```python
from build123d import *

# Parameters (mm, degrees)
SKETCH1_W           = 47
SKETCH1_H           = 78
SKETCH1_W_2         = 43
SKETCH1_H_2         = 74
EXTRUDE_THIN1_DEPTH = 15
SKETCH6_W           = 47
SKETCH6_H           = 78
BOSS_EXTRUDE1_DEPTH = 2
SKETCH8_W           = 43
SKETCH8_H           = 31
CUT_EXTRUDE1_DEPTH  = 10
CUT_EXTRUDE2_DEPTH  = 10
CUT_EXTRUDE3_DEPTH  = 10
CIRPATTERN1_COUNT   = 4
SKETCH12_R          = 1.6
CUT_EXTRUDE4_DEPTH  = 10
FILLET1_R           = 2


with BuildPart() as part:
    # Sketch1 → Extrude-Thin1 (new body)
    with BuildSketch(Plane.XY):
        with Locations((55.076537335, -3.402525622)):
            Rectangle(SKETCH1_W, SKETCH1_H)
        with Locations((55.076537335, -3.402525622)):
            Rectangle(SKETCH1_W_2, SKETCH1_H_2, mode=Mode.SUBTRACT)
    extrude(amount=EXTRUDE_THIN1_DEPTH)

    # Sketch6 → Boss-Extrude1 (add)
    with BuildSketch(Plane.XY.offset(15)):
        with Locations((55.076537335, -3.402525622)):
            Rectangle(SKETCH6_W, SKETCH6_H)
    extrude(amount=BOSS_EXTRUDE1_DEPTH)

    # Sketch8 → Cut-Extrude1 (cut)
    with BuildSketch(Plane(origin=(0, 0, 15), x_dir=(-1, 0, 0), z_dir=(0, 0, -1))):
        with Locations((-55.076537335, 18.097474378)):
            Rectangle(SKETCH8_W, SKETCH8_H)
    extrude(amount=-CUT_EXTRUDE1_DEPTH, mode=Mode.SUBTRACT)

    # Sketch9 → Cut-Extrude2 (cut)
    with BuildSketch(Plane(origin=(0, 0, 15), x_dir=(-1, 0, 0), z_dir=(0, 0, -1))):
        with BuildLine():
            ThreePointArc((-43.076537335, -18.902525622), (-43.989982945, -14.310324434), (-46.591255961, -10.417244248))
            Line((-46.591255961, -10.417244248), (-63.56181871, -27.387806996))
            ThreePointArc((-63.56181871, -27.387806996), (-50.484336147, -29.989080012), (-43.076537335, -18.902525622))
        make_face()
        with BuildLine():
            Line((-63.56181871, -27.387806996), (-46.591255961, -10.417244248))
            ThreePointArc((-46.591255961, -10.417244248), (-63.56181871, -10.417244248), (-63.56181871, -27.387806996))
        make_face()
    extrude(amount=-CUT_EXTRUDE2_DEPTH, mode=Mode.SUBTRACT)

    # Sketch11 → Cut-Extrude3 (cut)
    with BuildSketch(Plane(origin=(0, 0, 15), x_dir=(-1, 0, 0), z_dir=(0, 0, -1))):
        with BuildLine():
            ThreePointArc((-38.069685624, -3.395673911), (-38.183866325, -2.821648762), (-38.509025452, -2.335013739))
            Line((-38.509025452, -2.335013739), (-40.630345796, -4.456334083))
            ThreePointArc((-40.630345796, -4.456334083), (-38.995660475, -4.78149321), (-38.069685624, -3.395673911))
        make_face()
        with BuildLine():
            Line((-40.630345796, -4.456334083), (-38.509025452, -2.335013739))
            ThreePointArc((-38.509025452, -2.335013739), (-40.630345796, -2.335013739), (-40.630345796, -4.456334083))
        make_face()
    cut_extrude3 = extrude(amount=-CUT_EXTRUDE3_DEPTH, mode=Mode.SUBTRACT)

    # CirPattern1: Cut-Extrude3 ×4 about axis
    cirpattern1_axis = Axis((55.076537335, -18.902525622, 0), (0, 0, 1))
    for i in range(1, CIRPATTERN1_COUNT):
        add(cut_extrude3.rotate(cirpattern1_axis, i * 360 / CIRPATTERN1_COUNT), mode=Mode.SUBTRACT)

    # Sketch12 → Cut-Extrude4 (cut)
    with BuildSketch(Plane(origin=(0, 35.597474378, 0), x_dir=(1, 0, 0), z_dir=(0, 1, 0))):
        with BuildLine():
            ThreePointArc((55.076537335, -5.875), (52.451537335, -8.5), (55.076537335, -11.125))
            Line((55.076537335, -11.125), (55.076537335, -5.875))
        make_face()
        with BuildLine():
            Line((55.076537335, -5.875), (55.076537335, -11.125))
            ThreePointArc((55.076537335, -11.125), (56.932692636, -10.356155301), (57.701537335, -8.5))
            ThreePointArc((57.701537335, -8.5), (56.932692636, -6.643844699), (55.076537335, -5.875))
        make_face()
        with Locations(Location((43.446537335, -8.5, 0), (0, 0, 270))):
            Circle(SKETCH12_R)
        with Locations(Location((66.706537335, -8.5, 0), (0, 0, 270))):
            Circle(SKETCH12_R)
    extrude(amount=-CUT_EXTRUDE4_DEPTH, mode=Mode.SUBTRACT)

    # Fillet1
    fillet1_edges = [part.edges().sort_by_distance(p)[0] for p in [
        (33.576537335, 33.597474378, 8.5),
        (76.576537335, 33.597474378, 8.5),
    ]]
    fillet(fillet1_edges, radius=FILLET1_R)


solid = part.part
```
Geometry: final body of the model. Coordinates: model frame, mm. A direction names the side the tool comes from. Coordinates: 2 decimals unless noted, no trailing zeros. Loops run counter-clockwise (first coordinate to the right, second up) from the corner with the lowest first, then second, coordinate; pieces in that order, holes last. Notation, with made-up numbers: (59, 50.5) -> (115, 50.5) arc R14 cw to (115, 57.5) -> close; hole circle Ø3 at (27, -14.75). An arc over 180 degrees is marked (long way). Use a Markdown table: item, result. Add a question column.
(1) Section query B-B, the plane z = 2.5. Return loops of the section in (x, y), plus the area to 3 significant figures.
(2) Section query A-A, the plane y = 7. Return loops of the section in (x, z), plus the area to 3 significant figures.
(3) Section query D-D, the plane y = -12. Return loops of the section in (x, z), plus the area to 3 significant figures.
(4) Mould query, pull axis Y, two halves, no side actions, for faces 1 (the cylindrical face through (66.78, 34.61, 6.9)), 2 (the flat face through (55, -42.403, 8)), 3 (the cylindrical face through (76, 33, 9)), 4 (the flat face through (55, 35.597, 5)). Classes: pulls with the +Y half, pulls with the -Y half, needs draft (parallel to the pull), parting line crosses it, or undercut.
(5) Line query: line 1 along X through (y, z) = (35, 8.5); line 2 along Y through (x, z) = (58.5, 13); line 3 along X through (y, z) = (26.5, 13.5). Output: solid intervals per line, ascending.
(6) Access query for faces 5 (the flat face through (64, -28, 15)), 6 (the cylindrical face through (45.033, 34.611, 8.292)), 7 (the flat face through (55, 33.597, 5)). Directions: +Z, -Z, +X, -X, +Y, -Y. A direction counts if a zero-diameter tool reaches every point of the face in a straight line with its end or side. Return the directions, or none.
(7) Section query C-C, the plane x = 59. Return loops of the section in (y, z), plus the area to 3 significant figures.
Answer:
| question | item | result |
|---|---|---|
| 1 | outline | (31.58, -42.4) -> (78.58, -42.4) -> (78.58, 35.6) -> (31.58, 35.6) -> close; hole (33.58, -40.4) -> (76.58, -40.4) -> (76.58, 31.6) arc R2 ccw to (74.58, 33.6) -> (35.58, 33.6) arc R2 ccw to (33.58, 31.6) -> close |
| 1 | area | 486 mm^2 |
| 2 | outline | (31.58, 0) -> (33.58, 0) -> (33.58, 17) -> (31.58, 17) -> close; (76.58, 0) -> (78.58, 0) -> (78.58, 17) -> (76.58, 17) -> close |
| 2 | area | 68.0 mm^2 |
| 3 | outline | (31.58, 0) -> (33.58, 0) -> (33.58, 15) -> (45.26, 15) -> (45.26, 17) -> (31.58, 17) -> close; (64.89, 15) -> (76.58, 15) -> (76.58, 0) -> (78.58, 0) -> (78.58, 17) -> (64.89, 17) -> close |
| 3 | area | 115 mm^2 |
| 4 | face 1 | needs draft |
| 4 | face 2 | pulls with the -Y half |
| 4 | face 3 | undercut |
| 4 | face 4 | pulls with the +Y half |
| 5 | line 1 | x = 31.58 to 41.85, 45.05 to 52.45, 57.7 to 65.11, 68.31 to 78.58 |
| 5 | line 2 | y = -42.4 to -40.4, 33.6 to 35.6 |
| 5 | line 3 | x = 31.58 to 33.58, 76.58 to 78.58 |
| 6 | face 5 | -Z |
| 6 | face 6 | +Y |
| 6 | face 7 | +Z, -Z |
| 7 | outline | (-42.4, 0) -> (-40.4, 0) -> (-40.4, 15) -> (-30.24, 15) -> (-30.24, 17) -> (-42.4, 17) -> close; (-7.56, 15) -> (2.6, 15) -> (2.6, 17) -> (-7.56, 17) -> close; (33.6, 0) -> (35.6, 0) -> (35.6, 17) -> (33.6, 17) -> close |
| 7 | area | 109 mm^2 |
